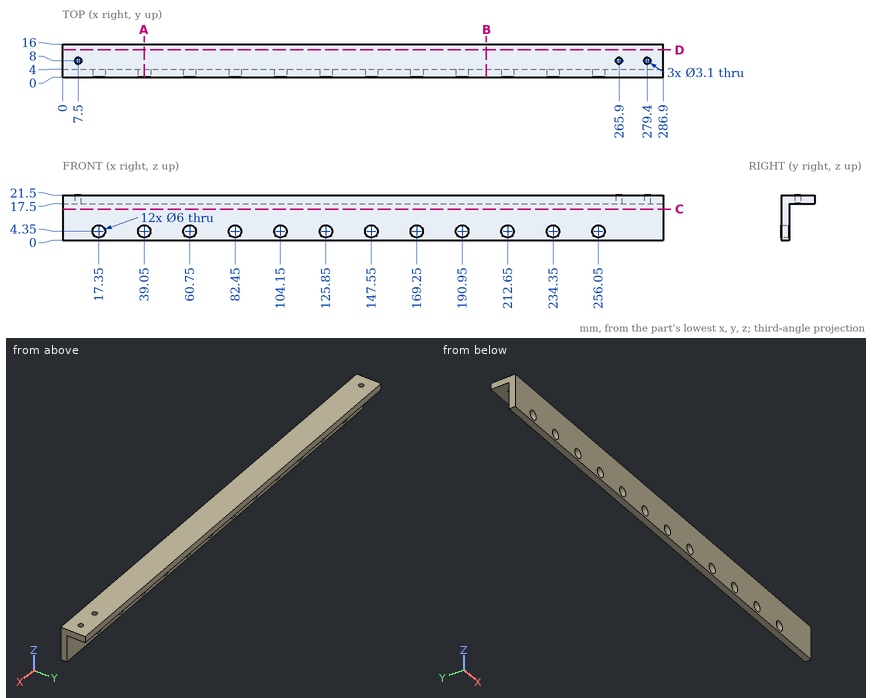
Job drawing, mm, ordinate dimensions from the low corner. One solid piece. Round coordinates to 2 decimals unless told otherwise and drop trailing zeros. Write each loop counter-clockwise with the first axis right and the second up, starting at its lowest first coordinate (ties: lowest second). Pieces come first, ordered by that corner, then holes. Notation, with made-up numbers: (-38, 30) -> (-2, 30) arc R27 cw to (-2, 49) -> close; hole circle Ø1 at (9, 32). An arc over 180 degrees is marked (long way). Answer as a JSON object with one key per item and string values.
(1) Band-saw the part on C-C, the plane z = 15. List the corners of the cut face in (x, y).
Reported:
{"outline": "(0, 0) -> (286.9, 0) -> (286.9, 4) -> (0, 4) -> close"}
(2) Probe probe 1 along Z at (x, y) = (104.15, 3.1); probe 2 along Z at (x, y) = (200.5, 14.75); probe 3 along Y at (x, z) = (125, 10.5). List the from-to ranges inside material, lowest first. Write a range as [from, to].
Reported:
{"probe 1": "z = [0, 1.35], [7.35, 21.5]", "probe 2": "z = [17.5, 21.5]", "probe 3": "y = [0, 4]"}
(3) Band-saw the part on D-D, the plane y = 13.25. List the corners of the cut face in (x, z).
Reported:
{"outline": "(0, 17.5) -> (286.9, 17.5) -> (286.9, 21.5) -> (0, 21.5) -> close"}
(4) Pin check, flat tips, straight feed: P1, Ø5.5, axis at x = 60.75, z = 4.35, coming from the +Y side; P2, Ø9.5, axis at x = 104.15, z = 4.35, coming from the +Y side; P3, Ø9.5, axis at x = 178.5, y = 10, coming from the -Z side. Stop position of each tip, or through.
Reported:
{"P1": "passes through", "P2": "stops at y = 4", "P3": "stops at z = 17.5"}
(5) Band-saw the part on A-A, the plane x = 39.05. List the corners of the cut face in (y, z), then the cut area to 3 significant figures.
Reported:
{"outline": "(0, 0) -> (4, 0) -> (4, 1.35) -> (0, 1.35) -> close; (0, 7.35) -> (4, 7.35) -> (4, 17.5) -> (16, 17.5) -> (16, 21.5) -> (0, 21.5) -> close", "area": "110 mm^2"}
(6) Band-saw the part on B-B, the plane x = 202.5. List the corners of the cut face in (y, z), then the cut area to 3 significant figures.
Reported:
{"outline": "(0, 0) -> (4, 0) -> (4, 17.5) -> (16, 17.5) -> (16, 21.5) -> (0, 21.5) -> close", "area": "134 mm^2"}
